Here's the drawing with two shaded views (mm, measured from the low corner). I have some questions. A direction names the side the tool comes from. Give positions to 0.01 mm unless a question says otherwise; leave off trailing zeros. Write each loop counter-clockwise with the first axis right and the second up, starting at its lowest first coordinate (ties: lowest second). Pieces come first, ordered by that corner, then holes. Notation, with made-up numbers: M 30.25,-14.75 L 61.25,-14.75 A17 ccw 61.25,16.25 Z; hole C -35.5,22.5 d9. An arc over 180 degrees is marked long. Answer as a JSON object with one key per item and string values. Group by question number.
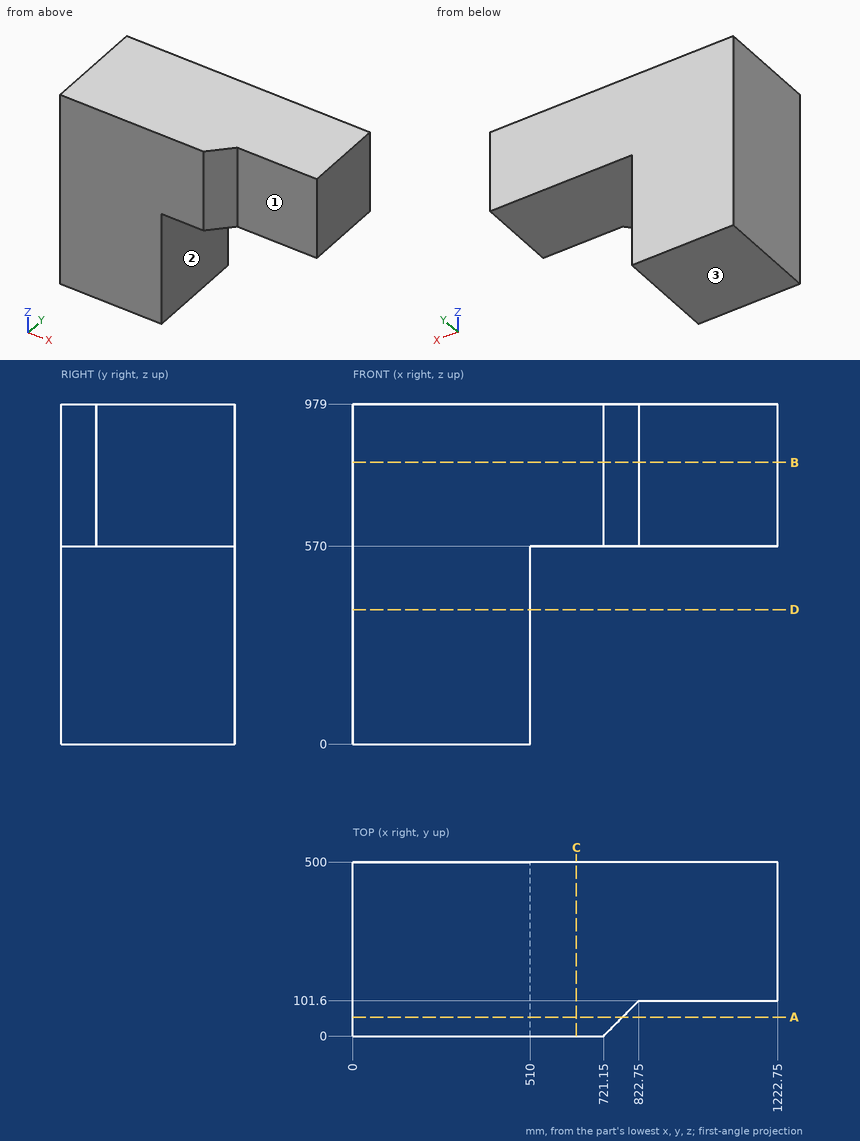
1) If we section it at B-B, the plane z = 811: List the corners of the cut face in (x, y) for me, plus the area to 3 significant figures.
2) Please list where these lines run through material, in increasing order: line 1 along X through (y, z) = (424.5, 550.5); line 2 along Z through (x, y) = (585, 423); line 3 along Y through (x, z) = (846, 618). Write a range as from..to.
3) If we section it at D-D, the plane z = 387.5: List the corners of the cut face in (x, y) for me.
4) If we section it at C-C, the plane x = 643: List the corners of the cut face in (y, z) for me, plus the area to 4 significant figures.
5) I'm going to push a flat-ended pin straight in: pin 1 (8 mm diameter, centred on y = 430.5, z = 194.5, fed in from +X). Where does the tip first touch, or does it pass through?
6) For the marked faces 1, 2 and 3, which set-ups out of +Z, -Z, +X, -X, +Y, -Y let a thin tool reach every point of the face, with its end or its side?
7) If we section it at A-A, the plane y = 54: List the corners of the cut face in (x, z) for me.
Taken from the geometry:
{
 "1": {"outline": "M 0,0 L 721.15,0 L 822.75,101.6 L 1222.75,101.6 L 1222.75,500 L 0,500 Z", "area": "566,000 mm²"},
 "2": {"line 1": "0..510", "line 2": "570..979", "line 3": "101.6..500"},
 "3": {"outline": "M 0,0 L 510,0 L 510,500 L 0,500 Z"},
 "4": {"outline": "M 0,570 L 500,570 L 500,979 L 0,979 Z", "area": "204,500 mm²"},
 "5": {"pin 1": "x = 510"},
 "6": {"face 1": "+Z, -Z, +X, -Y", "face 2": "-Z, +X, +Y, -Y", "face 3": "-Z, +X, -X, +Y, -Y"},
 "7": {"outline": "M 0,0 L 510,0 L 510,570 L 775.15,570 L 775.15,979 L 0,979 Z"}
}
